from build123d import *

# Parameters (mm, degrees)
F0_W     = 40
F0_H     = 35
F1_DEPTH = 5
F2_W     = 35
F2_H     = 35
F3_DEPTH = 3
F4_SIZE  = 0.5


with BuildPart() as f1:
    # F0 (on Top) → F1 (new body)
    with BuildSketch(Plane.XY):
        with Locations((20, 17.5)):
            Rectangle(F0_W, F0_H)
    extrude(amount=F1_DEPTH)

    # F2 (on face) → F3 (cut)
    with BuildSketch(Plane.XY.offset(5)):
        with Locations((22.5, 17.5)):
            Rectangle(F2_W, F2_H)
    extrude(amount=-F3_DEPTH, mode=Mode.SUBTRACT)

    # F4
    f4_edges = [f1.edges().sort_by_distance(p)[0] for p in [
        (2.5, 35, 5),
        (5, 17.5, 5),
        (2.5, 0, 5),
        (0, 17.5, 5),
        (20, 0, 0),
        (40, 0, 1),
        (22.5, 0, 2),
        (5, 0, 3.5),
        (0, 0, 2.5),
        (20, 35, 0),
        (0, 35, 2.5),
        (5, 35, 3.5),
        (22.5, 35, 2),
        (40, 35, 1),
    ]]
    chamfer(f4_edges, length=F4_SIZE)


solid = f1.part
The model under review builds one solid part; all positions refer to its coordinate system, in mm. A direction names the side the tool comes from. Coordinates: 2 decimals unless noted, no trailing zeros. Loops run counter-clockwise (first coordinate to the right, second up) from the corner with the lowest first, then second, coordinate; pieces in that order, holes last.
(1) Consider section A-A, the plane x = 29. Give the boundary of the cut face in (y, z), plus the area to 3 significant figures.
Determined:
outline: (0, 0.5) - (0.5, 0) - (34.5, 0) - (35, 0.5) - (35, 1.5) - (34.5, 2) - (0.5, 2) - (0, 1.5) - close
area: 69.5 mm2
(2) Wall thickness on L1, parallel to Z at x = 13, y = 14; L2, parallel to X at y = 8, z = 3.7: over which ranges is each line inside the solid? List them lowest first.
Determined:
L1: z = 0 to 2
L2: x = 0 to 5
(3) Consider section B-B, the plane y = 25. Give the boundary of the cut face in (x, z).
Determined:
outline: (0, 0) - (40, 0) - (40, 2) - (5, 2) - (5, 4.5) - (4.5, 5) - (0.5, 5) - (0, 4.5) - close
(4) Insertion check: P1, Ø5, axis at x = 10.5, y = 16, coming from the +Z side; P2, Ø0.8, axis at y = 25, z = 3, coming from the +X side. Each pin has a flat end and moves straight along its axis. Give the tip position at first contact, or say it passes through.
Determined:
P1: stops at z = 2
P2: stops at x = 5
(5) Tool access review of faces 1 (the flat face through (16, 0, 1)), 2 (the flat face through (5, 17, 3)): name each direction out of +Z, -Z, +X, -X, +Y, -Y from which nothing blocks a thin tool from reaching the whole face with its end or side.
Determined:
face 1: +Z, -Z, +X, -X, -Y
face 2: +Z, +X, +Y, -Y
